CAD build for the part. Positions are in the model's coordinates, mm. Face numbers are marked on the shaded views. A direction names the side the tool comes from. Round coordinates to 2 decimals unless told otherwise and drop trailing zeros. Write each loop counter-clockwise with the first axis right and the second up, starting at its lowest first coordinate (ties: lowest second). Pieces come first, ordered by that corner, then holes. Notation, with made-up numbers: (-14, -32) -> (14, -32) arc R21 ccw to (14, -11) -> close; hole circle Ø9 at (78, -29.5). An arc over 180 degrees is marked (long way). Answer in a Markdown table with one row per item. Add a question column.
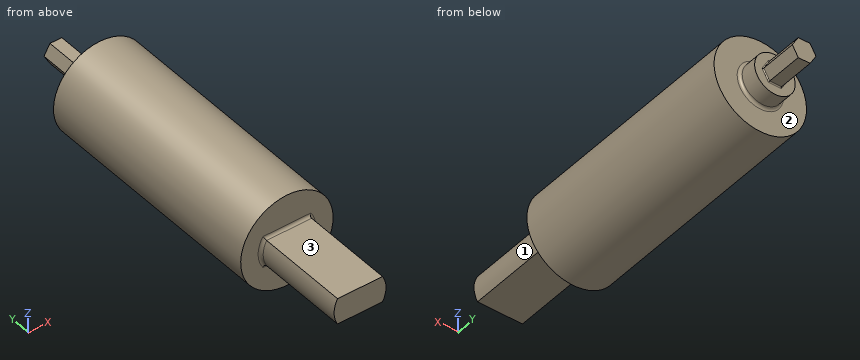
```python
from build123d import *

# Parameters (mm, degrees)
CROQUIS5_R              = 4.9
SALIENTE_EXTRUIR1_DEPTH = 35.6
CROQUIS6_R              = 2.15
SALIENTE_EXTRUIR2_DEPTH = 2
SALIENTE_EXTRUIR3_DEPTH = 4
REDONDEO3_R             = 0.1
REDONDEO4_R             = 0.3
CORTAR_EXTRUIR1_START   = -10
CROQUIS8_R              = 4.9
CORTAR_EXTRUIR1_DEPTH   = 10
REDONDEO5_R             = 0.3


with BuildPart() as part:
    # Croquis5 → Saliente-Extruir1 (new body)
    with BuildSketch(Plane(origin=(0, 0, 0), x_dir=(1, 0, 0), z_dir=(0, 1, 0))):
        with Locations(Location((0, 0, 0), (0, 0, 270))):
            Circle(CROQUIS5_R)
    extrude(amount=-SALIENTE_EXTRUIR1_DEPTH)

    # Croquis6 → Saliente-Extruir2 (add)
    with BuildSketch(Plane(origin=(0, 0, 0), x_dir=(1, 0, 0), z_dir=(0, 1, 0))):
        with Locations(Location((0, 0, 0), (0, 0, 270))):
            Circle(CROQUIS6_R)
    extrude(amount=SALIENTE_EXTRUIR2_DEPTH)

    # Croquis7 → Saliente-Extruir3 (add)
    with BuildSketch(Plane(origin=(0, 2, 0), x_dir=(1, 0, 0), z_dir=(0, 1, 0))):
        Polygon((1.252850084, 0), (0.626425042, 1.085), (-0.626425042, 1.085), (-1.252850084, 0), (-0.626425042, -1.085), (0.626425042, -1.085), align=None)
    extrude(amount=SALIENTE_EXTRUIR3_DEPTH)

    # Redondeo3
    redondeo3_edges = [part.edges().sort_by_distance(p)[0] for p in [
        (0.939637563, 2, 0.5425),
        (0.939637563, 2, -0.5425),
        (0, 2, -1.085),
        (-0.939637563, 2, -0.5425),
        (-0.939637563, 2, 0.5425),
        (0, 2, 1.085),
    ]]
    fillet(redondeo3_edges, radius=REDONDEO3_R)

    # Redondeo4
    redondeo4_edges = [part.edges().sort_by_distance(p)[0] for p in [
        (0, 0, -2.15),
    ]]
    fillet(redondeo4_edges, radius=REDONDEO4_R)

    # Croquis8 → Cortar-Extruir1 (cut)
    with BuildSketch(Plane.XZ.offset(35.6).offset(CORTAR_EXTRUIR1_START)):
        with Locations(Location((0, 0, 0), (0, 0, 90))):
            Circle(CROQUIS8_R)
        with BuildLine():
            ThreePointArc((-2.38156986, 1.375), (-2.75, 0), (-2.38156986, -1.375))
            Line((-2.38156986, -1.375), (2.38156986, -1.375))
            ThreePointArc((2.38156986, -1.375), (2.75, 0), (2.38156986, 1.375))
            Line((2.38156986, 1.375), (-2.38156986, 1.375))
        make_face(mode=Mode.SUBTRACT)
    extrude(amount=CORTAR_EXTRUIR1_DEPTH, mode=Mode.SUBTRACT)

    # Redondeo5
    redondeo5_edges = [part.edges().sort_by_distance(p)[0] for p in [
        (0, -25.6, 1.375),
        (-2.75, -25.6, 0),
        (0, -25.6, -1.375),
        (2.75, -25.6, 0),
    ]]
    fillet(redondeo5_edges, radius=REDONDEO5_R)


solid = part.part
```
Item 1: Saw through at C-C on z = -3. Give the cut face in (x, y), then the cut area to 3 significant figures.
Item 2: Pin check, flat tips, straight feed: pin 1 (1 mm diameter, centred on x = 2.5, y = -24, fed in from -Z); pin 2 (3 mm diameter, centred on x = -3, y = -5, fed in from -Z); pin 3 (1.4 mm diameter, centred on x = 0, y = 4.5, fed in from +Z) (3 decimals). Stop position of each tip, or through.
Item 3: Drill centre lines: probe 1 along Y at (x, z) = (-2.5, 0.25); probe 2 along Y at (x, z) = (-3, -0.75); probe 3 along Z at (x, y) = (1.5, -26.5) (3 decimals). Where is each one in solid material? Low to high.
Item 4: Saw through at A-A on x = 0. Give the cut face in (y, z) (3 decimals).
Item 5: Saw through at D-D on y = -31.5. Give the cut face in (x, z) (3 decimals).
Item 6: Tool access for the marked faces 1, 2 and 3: list every direction of +Z, -Z, +X, -X, +Y, -Y with a clear straight run to the whole face (end or side of a thin tool).
Item 7: Saw through at B-B on y = -14.5. Give the cut face in (x, z).
Recorded:
| question | item | result |
|---|---|---|
| 1 | outline | (-3.87, -25.6) -> (3.87, -25.6) -> (3.87, 0) -> (-3.87, 0) -> close |
| 1 | area | 198 mm2 |
| 2 | pin 1 | z = -4.47 |
| 2 | pin 2 | z = -4.66 |
| 2 | pin 3 | z = 1.085 |
| 3 | probe 1 | -35.6 to 0 |
| 3 | probe 2 | -25.6 to 0 |
| 3 | probe 3 | -1.375 to 1.375 |
| 4 | outline | (-35.6, -1.375) -> (-25.9, -1.375) arc R0.3 cw to (-25.6, -1.675) -> (-25.6, -4.9) -> (0, -4.9) -> (0, -2.45) arc R0.3 cw to (0.3, -2.15) -> (2, -2.15) -> (2, -1.185) arc R0.1 cw to (2.1, -1.085) -> (6, -1.085) -> (6, 1.085) -> (2.1, 1.085) arc R0.1 cw to (2, 1.185) -> (2, 2.15) -> (0.3, 2.15) arc R0.3 cw to (0, 2.45) -> (0, 4.9) -> (-25.6, 4.9) -> (-25.6, 1.675) arc R0.3 cw to (-25.9, 1.375) -> (-35.6, 1.375) -> close |
| 5 | outline | (-2.382, -1.375) -> (2.382, -1.375) arc R2.75 ccw to (2.382, 1.375) -> (-2.382, 1.375) arc R2.75 ccw to start |
| 6 | face 1 | +X, -Y |
| 6 | face 2 | +Y |
| 6 | face 3 | +Z, +X, -X, -Y |
| 7 | outline | circle Ø9.8 at (0, 0) |
